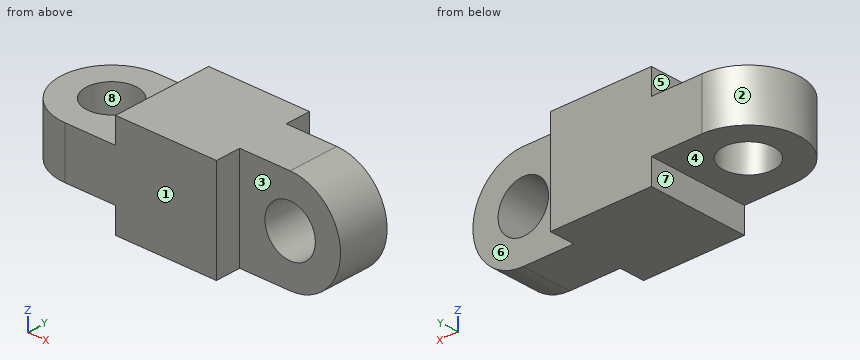
from build123d import *

# Parameters (mm, degrees)
ESQUISSE1_R        = 5
BOSS_EXTRU_1_DEPTH = 20
ESQUISSE2_R        = 5
BOSS_EXTRU_2_DEPTH = 20


with BuildPart() as part:
    # Esquisse1 → Boss.-Extru.1 (new body)
    with BuildSketch(Plane.XY):
        with BuildLine():
            Line((50, 5), (50, 15))
            Line((50, 15), (30, 15))
            Line((30, 15), (30, 20))
            Line((30, 20), (0, 20))
            ThreePointArc((0, 20), (-10, 10), (0, 0))
            Line((0, 0), (30, 0))
            Line((30, 0), (30, 5))
            Line((30, 5), (50, 5))
        make_face()
        with Locations((0, 10)):
            Circle(ESQUISSE1_R, mode=Mode.SUBTRACT)
    extrude(amount=BOSS_EXTRU_1_DEPTH)


with BuildPart() as body_2:
    # Esquisse2 → Boss.-Extru.2 (new body)
    with BuildSketch(Plane(origin=(0, 0, 0), x_dir=(1, 0, 0), z_dir=(0, 1, 0))):
        with BuildLine():
            Line((-10, -5), (-10, -15))
            Line((-10, -15), (10, -15))
            Line((10, -15), (10, -20))
            Line((10, -20), (40, -20))
            ThreePointArc((40, -20), (50, -10), (40, 0))
            Line((40, 0), (10, 0))
            Line((10, 0), (10, -5))
            Line((10, -5), (-10, -5))
        make_face()
        with Locations((40, -10)):
            Circle(ESQUISSE2_R, mode=Mode.SUBTRACT)
    extrude(amount=BOSS_EXTRU_2_DEPTH)

    # Combiner1: intersect part
    add(part.part, mode=Mode.INTERSECT)


solid = body_2.part
The model under review builds one solid part; all positions refer to its coordinate system, in mm. Face numbers are marked on the shaded views. A direction names the side the tool comes from. Round coordinates to 2 decimals unless told otherwise and drop trailing zeros. Loops run counter-clockwise (first coordinate to the right, second up) from the corner with the lowest first, then second, coordinate; pieces in that order, holes last. Notation, with made-up numbers: (55, 81) -> (61, 81) arc R10 ccw to (61, 86) -> close; hole circle Ø6 at (21.25, -14). An arc over 180 degrees is marked (long way). Return JSON: item names as keys, results as strings.
(1) Add section B-B on y = 7. Write out the cut boundary in (x, z), plus the area to 3 significant figures.
Solved:
{"outline": "(-9.54, 5) -> (-4, 5) -> (-4, 15) -> (-9.54, 15) -> close; (4, 5) -> (10, 5) -> (10, 0) -> (40, 0) arc R10 ccw to (40, 20) -> (10, 20) -> (10, 15) -> (4, 15) -> close; hole circle Ø10 at (40, 10)", "area": "794 mm2"}
(2) For line 1 (Y direction, x = 0, z = 11); line 2 (X direction, y = 10, z = 12); line 3 (X direction, y = 12.75, z = 5.5), list the stretches that pass through material, from the lowest coordinate up.
Solved:
{"line 1": "0 to 5, 15 to 20", "line 2": "-10 to -5, 5 to 35.42, 44.58 to 49.8", "line 3": "-9.61 to -4.18, 4.18 to 37.82, 42.18 to 48.93"}
(3) Add section D-D on x = 31.5. Write out the cut boundary in (y, z), plus the area to 3 significant figures.
Solved:
{"outline": "(5, 0) -> (15, 0) -> (15, 20) -> (5, 20) -> close", "area": "200 mm2"}
(4) Add section A-A on z = 10. Write out the cut boundary in (x, y).
Solved:
{"outline": "(0, 0) -> (30, 0) -> (30, 5) -> (35, 5) -> (35, 15) -> (30, 15) -> (30, 20) -> (0, 20) arc R10 ccw to start; (45, 5) -> (50, 5) -> (50, 15) -> (45, 15) -> close; hole circle Ø10 at (0, 10)"}
(5) For pin 1 (6 mm diameter, centred on x = 36, z = 15, fed in from +Y); pin 2 (10 mm diameter, centred on x = 1, y = 7, fed in from +Z); pin 3 (6 mm diameter, centred on x = 43.5, z = 7.5, fed in from -Y); pin 4 (8 mm diameter, centred on x = 40, z = 10, fed in from -Y), all flat-tipped, find the tip position at first contact; note any pin that passes through.
Solved:
{"pin 1": "y = 15", "pin 2": "z = 15", "pin 3": "y = 5", "pin 4": "through"}
(6) The part is to be moulded in two halves that separate along Y. For the marked faces 6, 7 and 8, say which applies: released by +Y, released by -Y, zero draft, split by the parting line, or undercut.
Solved:
{"face 6": "released by +Y", "face 7": "zero draft", "face 8": "undercut"}
(7) Add section C-C on z = 18.5. Write out the cut boundary in (x, y), plus the area to 3 significant figures.
Solved:
{"outline": "(10, 0) -> (30, 0) -> (30, 5) -> (45.27, 5) -> (45.27, 15) -> (30, 15) -> (30, 20) -> (10, 20) -> close", "area": "553 mm2"}
(8) For the marked faces 1, 2, 3, 4 and 5, list the 3-axis set-ups (+Z, -Z, +X, -X, +Y, -Y) from which the entire face can be reached by the end or side of a thin tool; tool diameter is ignored.
Solved:
{"face 1": "+Z, -Z, +X, -X, -Y", "face 2": "+Z, -Z, -X", "face 3": "+Z, -Z, +X, -Y", "face 4": "-Z, -X, +Y, -Y", "face 5": "+Z, -X, +Y, -Y"}
